Verification items for the finished model (mm, model axes). Face numbers are marked on the shaded views. A direction names the side the tool comes from. Coordinates: 2 decimals unless noted, no trailing zeros. Order: outer loops, then holes, each group sorted by start corner. A loop starts at its lowest first (then second) coordinate and runs counter-clockwise, first axis right, second up. Notation, with made-up numbers: M 16,77 L 64,77 A10 ccw 64,92 Z; hole C 72,50 d4. An arc over 180 degrees is marked long. Return JSON: item names as keys, results as strings. Group by question number.
Q1. Mould release check, pull along X, two halves, no side actions. Record for the marked faces 1, 2, 3 and 4: pulls with the +X half, pulls with the -X half, needs draft (parallel to the pull), parting line crosses it, or undercut.
Q2. Section check C-C, the plane z = 25. Enter the section's corners in (x, y) (3 decimals).
Q3. Access from +Z, -Z, +X, -X, +Y, -Y to the whole of each face (thin tool, end or side, straight path). Record for the marked faces 5, 6, 7 and 8.
Q4. Go/stop test with flat-tipped pins: pin 1 Ø6 at (x, z) = (7, 35.5) entering from +Y; pin 2 Ø0.6 at (x, y) = (-0.5, 2.5) entering from -Z; pin 3 Ø4 at (x, y) = (8.5, 13) entering from -Z. Record where each tip stops, or that it passes through.
Q5. Section check A-A, the plane y = 11.25. Enter the section's corners in (x, z) (3 decimals), then the cut area to 3 significant figures.
Q6. Thickness scan on probe 1 along X at (y, z) = (14, 10.5) (3 decimals); probe 2 along X at (y, z) = (2.5, 5.5) (3 decimals); probe 3 along Y at (x, z) = (12, 29.5). Record the ranges inside material, lowest first.
Q7. Section check D-D, the plane y = 14. Enter the section's corners in (x, z) (1 decimal).
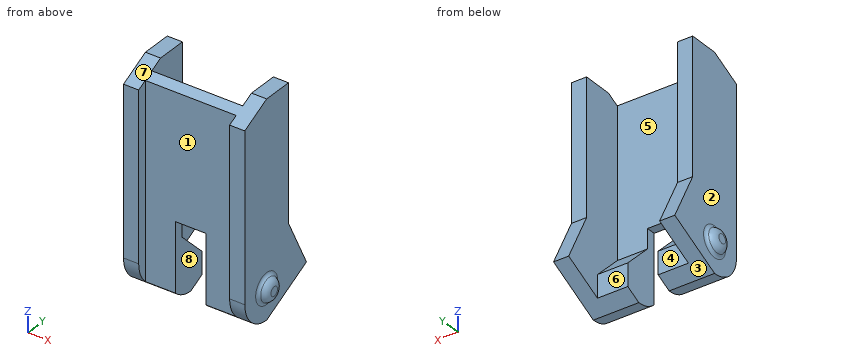
Autodesk Inventor part; units mm, degrees
ref_plane "YZ Plane" through (0, 0, 0) normal (1, 0, 0) x (0, 1, 0)
ref_plane "XZ Plane" through (0, 0, 0) normal (0, 1, 0) x (-1, 0, 0)
ref_plane "XY Plane" through (0, 0, 0) normal (0, 0, 1) x (1, 0, 0)
sketch "Sketch2" plane through (0, 0, 0) normal (1, 0, 0) x (0, 1, 0)
  line L0 (0, 0) -> (12.7, 0) construction
  line L1 (12.7, 0) -> (12.7, 44.45) construction
  line L2 (12.7, 44.45) -> (0, 44.45) construction
  line L3 (0, 44.45) -> (0, 0) construction
  arc A0 (0, 6.35) -> (6.35, 0) centre (6.35, 6.35) ccw
  line L4 (6.35, 0) -> (6.35, 44.45) construction
  line L5 (6.35, 44.45) -> (0, 41.275)
  line L6 (0, 41.275) -> (0, 6.35)
  line L7 (6.35, 44.45) -> (6.35, 42.545)
  line L8 (6.35, 42.545) -> (1.905, 40.3225)
  line L9 (1.905, 40.3225) -> (1.905, 9.525)
  line L10 (6.35, 44.45) -> (12.7, 44.45)
  line L11 (6.35, 0) -> (12.7, 3.175)
  line L12 (12.7, 3.175) -> (12.7, 44.45)
  line L13 (6.35, 6.35) -> (6.35, 0)
  line L14 (6.35, 6.35) -> (1.905, 9.525)
  circle A1 centre (6.35, 6.35) radius 2.54
  line L15 (0, 16.1925) -> (12.7, 16.1925)
  line L16 (3.81, 0.5301) -> (3.81, 43.18)
  line L17 (1.905, 9.525) -> (1.905, 1.8152)
  line L18 (1.905, 40.3225) -> (1.905, 42.2275)
  line L19 (12.7, 16.1925) -> (17.907, 5.7785)
  line L20 (12.7, 3.175) -> (17.907, 5.7785)
  dimension "d2" = 12.7
  dimension "d3" = 44.45
  dimension "d4" = 12.7
  dimension "d5" = 3.175
  dimension "d6" = 1.905
  dimension "d7" = 1.905
  dimension "d8" = 3.175
  dimension "d9" = 3.175
  dimension "d10" = 5.08
  dimension "d11" = 16.1925
  dimension "d22" = 1.905
extrude "Extrusion1" add sketch "Sketch2" along normal mid plane 28.575 contours A1 L14 L13 | L13 L14 A1
extrude "Extrusion2" add sketch "Sketch2" along normal mid plane 25.4
extrude "Extrusion4" cut sketch "Sketch2" along normal mid plane 6.35 contours L6 L15 L9 L17 A0 | L17 L14 L16 A0 | L16 A1 L13 A0 | L9 L15 L16 L14 | L13 A1 L14 L16 L15 L12 L11 | L16 L14 A1 | A1 L14 L13 | L13 L14 A1
fillet "Fillet1" radius 1.5875 2 edges at (-14.2875, 3.81, 6.35) (14.2875, 3.81, 6.35)
fillet "Fillet2" radius 0.7937 4 edges at (-12.7, 3.81, 6.35) (-12.7001, 3.81, 6.35) (12.7001, 3.81, 6.35) (12.7, 3.81, 6.35)
sketch "Sketch3" plane through (0, 0, 0) normal (1, 0, 0) x (0, 1, 0)
  line L0 (12.7, 44.45) -> (12.7, 16.1925)
  line L1 (17.907, 5.7785) -> (6.35, 0)
  arc A0 (0, 6.35) -> (6.35, 0) centre (6.35, 6.35) ccw
  line L2 (0, 6.35) -> (0, 41.275)
  line L3 (0, 41.275) -> (6.35, 44.45)
  line L4 (6.35, 44.45) -> (12.7, 44.45)
  circle A1 centre (6.35, 6.35) radius 3.1976
  circle A2 centre (6.35, 6.35) radius 3.1976
  line L5 (3.81, 0.5301) -> (3.81, 43.18)
  line L6 (1.905, 40.3225) -> (1.905, 9.525)
  line L7 (1.905, 42.2275) -> (1.905, 1.8152)
  line L8 (0, 0) -> (1.905, 0)
  line L9 (1.905, 0) -> (1.905, 42.2275)
  line L10 (1.905, 42.2275) -> (0, 42.2275)
  line L11 (0, 42.2275) -> (0, 0)
  circle A3 centre (6.35, 6.35) radius 3.1976
  line L12 (9.5476, 44.45) -> (9.5476, 1.5988)
  line L13 (12.7, 44.45) -> (9.5476, 44.45)
  line L14 (9.5476, 44.45) -> (9.5476, 0)
  line L15 (9.5476, 0) -> (12.7, 0)
  line L16 (12.7, 0) -> (12.7, 44.45)
  line L17 (6.3337, 9.5475) -> (1.905, 9.525)
  circle A4 centre (6.35, 6.35) radius 3.1976
  line L18 (9.5476, 6.35) -> (9.5476, 0)
  line L19 (9.5476, 0) -> (1.905, 0)
  line L20 (9.5476, 7.1442) -> (9.5476, 44.45)
  line L21 (6.35, 44.45) -> (3.81, 43.18)
  line L22 (3.81, 12.0876) -> (3.81, 43.18)
  line L23 (1.905, 42.2275) -> (6.35, 44.45)
  line L24 (6.35, 44.45) -> (9.5476, 44.45)
  line L25 (9.5476, 44.45) -> (9.5476, 6.35)
  line L26 (9.5476, 6.35) -> (1.905, 13.9926)
  line L27 (12.7, 16.1925) -> (17.907, 5.7785)
  dimension "d25" = 1.905
extrude "Extrusion6" cut sketch "Sketch3" along normal mid plane 19.05 contours L0 L16 L1 L12 L4 | L27 L1 L16 | L12 A1 L26 L5 L3 L4 | L26 A1 | L7 L6 A0 L2 L3
equation "\"d7\" = d6"
equation "\"d22\" = d7"
properties part number "LegV2"
Numbers:
{
 "1": {"face 1": "undercut", "face 2": "pulls with the -X half", "face 3": "needs draft", "face 4": "undercut"},
 "2": {"outline": "M -12.7,0 L -9.525,0 L -9.525,1.905 L 9.525,1.905 L 9.525,0 L 12.7,0 L 12.7,12.7 L 9.525,12.7 L 9.525,3.81 L -9.525,3.81 L -9.525,12.7 L -12.7,12.7 Z"},
 "3": {"face 5": "+Z, +Y", "face 6": "+Z, -Z, +Y", "face 7": "+Z, +X, -X, -Y", "face 8": "-Z, +Y, -Y"},
 "4": {"pin 1": "stops at y = 12.7", "pin 2": "stops at z = 16.19", "pin 3": "stops at z = 2.47"},
 "5": {"outline": "M -12.7,2.45 L -9.525,2.45 L -9.525,44.45 L -12.7,44.45 Z; M 9.525,2.45 L 12.7,2.45 L 12.7,44.45 L 9.525,44.45 Z", "area": "267 mm2"},
 "6": {"probe 1": "x = -12.7 to -9.525, 9.525 to 12.7", "probe 2": "x = -12.7 to -3.175, 3.175 to 12.7", "probe 3": "y = 0 to 12.7"},
 "7": {"outline": "M -12.7,3.8 L -9.5,3.8 L -9.5,13.6 L -12.7,13.6 Z; M 9.5,3.8 L 12.7,3.8 L 12.7,13.6 L 9.5,13.6 Z"}
}
